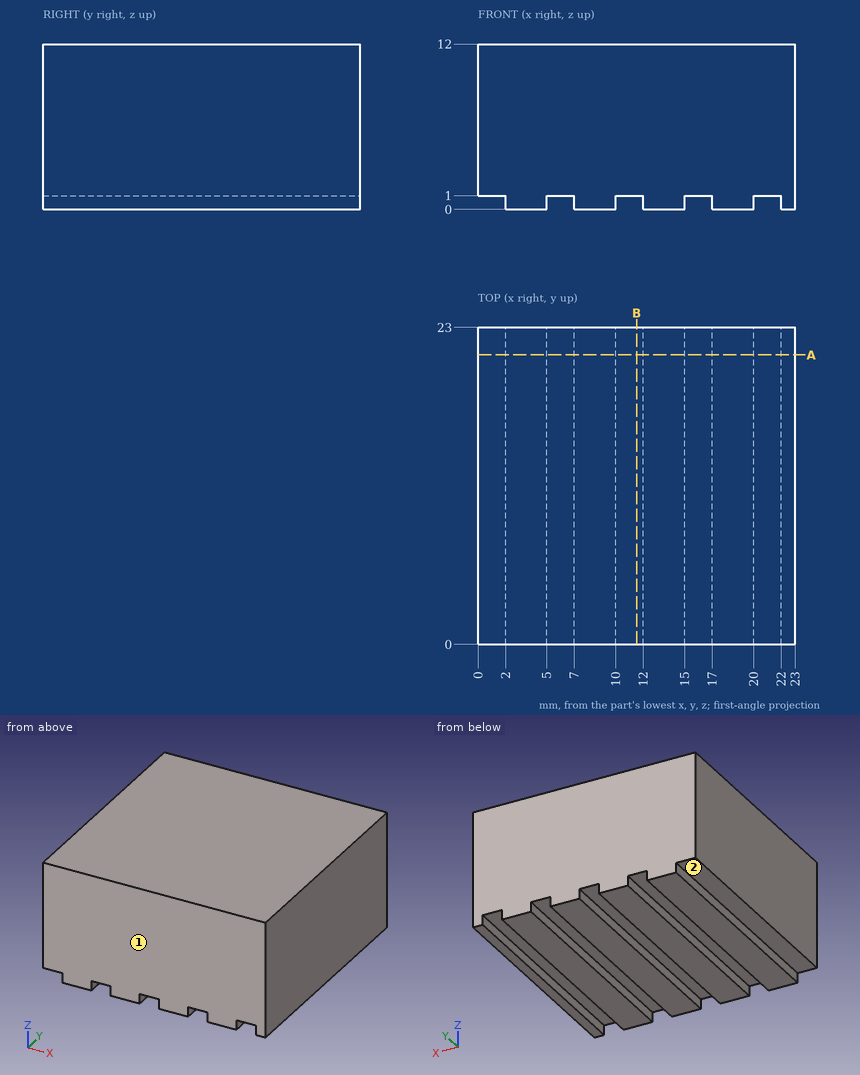
Can you work these out from the drawing? Everything is in mm from the part's minimum corner. A direction names the side the tool comes from. Round coordinates to 2 decimals unless told otherwise and drop trailing zeros. Loops run counter-clockwise (first coordinate to the right, second up) from the corner with the lowest first, then second, coordinate; pieces in that order, holes last. Notation, with made-up numbers: (-20, 45.25) - (-1, 45.25) arc R29 cw to (-1, 76.25) - close; hole circle Ø9 at (7, -16). An arc over 180 degrees is marked (long way). Answer in a Markdown table with one row per item. Add a question column.
Q1. Which directions (+Z, -Z, +X, -X, +Y, -Y) give clear straight access to the entire face, cutting with the end or side of a thin tool? Please do the marked faces 1 and 2.
Q2. I want a section at B-B on x = 11.5. List the corners of the cut face in (y, z) for me, and give its area (3 significant figures).
Q3. I want a section at A-A on y = 21. List the corners of the cut face in (x, z) for me, and give its area (3 significant figures).
Q4. I need wall thicknesses on L1, parallel to Z at x = 20.25, y = 9.5. Which ranges of the line are inside material? Lowest first, please.
Q5. For pin 1 Ø0.8 at (y, z) = (7.5, 0.5) entering from -X; pin 2 Ø0.6 at (x, y) = (16, 11) entering from -Z, each with a flat end and sliding along its axis, tell me the tip position at first contact or that it passes through.
A:
| question | item | result |
|---|---|---|
| 1 | face 1 | +Z, -Z, +X, -X, -Y |
| 1 | face 2 | -Z, -X, +Y, -Y |
| 2 | outline | (0, 1) - (23, 1) - (23, 12) - (0, 12) - close |
| 2 | area | 253 mm^2 |
| 3 | outline | (0, 1) - (2, 1) - (2, 0) - (5, 0) - (5, 1) - (7, 1) - (7, 0) - (10, 0) - (10, 1) - (12, 1) - (12, 0) - (15, 0) - (15, 1) - (17, 1) - (17, 0) - (20, 0) - (20, 1) - (22, 1) - (22, 0) - (23, 0) - (23, 12) - (0, 12) - close |
| 3 | area | 266 mm^2 |
| 4 | L1 | 1 to 12 |
| 5 | pin 1 | x = 2 |
| 5 | pin 2 | z = 1 |
